```python
from build123d import *

# Parameters (mm, degrees)
SKETCH1_R               = 94.996
SKETCH1_R_2             = 53.975
TOP_OF_HATCH_DEPTH      = 3.302
SKETCH2_R               = 94.996
SKETCH2_R_2             = 89.789
HATCH_BODY_DEPTH        = 259.08
SKETCH3_R               = 13.335
CHARGE_TUBE_HOLES_DEPTH = 263.382
SKETCH4_R               = 3.81
BOLT_HOLES_DEPTH        = 263.382
SKETCH_5_R              = 5.08
ANTENNA_HOLES_DEPTH     = 263.382
SKETCH5_R               = 3.81
SKETCH5_R_2             = 3.175
INNER_SCREW_HOLES_DEPTH = 263.382
SKETCH8_R               = 1.397
CUT_EXTRUDE1_DEPTH      = 190.992
CUT_EXTRUDE4_DEPTH      = 263.3820001


with BuildPart() as part:
    # Sketch1 → Top of Hatch (new body)
    with BuildSketch(Plane(origin=(0, 0, 0), x_dir=(1, 0, 0), z_dir=(0, 1, 0))):
        Circle(SKETCH1_R)
        Circle(SKETCH1_R_2, mode=Mode.SUBTRACT)
    extrude(amount=TOP_OF_HATCH_DEPTH)

    # Sketch2 → Hatch Body (add)
    with BuildSketch(Plane(origin=(0, 3.302, 0), x_dir=(1, 0, 0), z_dir=(0, 1, 0))):
        Circle(SKETCH2_R)
        Circle(SKETCH2_R_2, mode=Mode.SUBTRACT)
    extrude(amount=HATCH_BODY_DEPTH)

    # Sketch3 → Charge Tube Holes (cut, through all)
    with BuildSketch(Plane.XZ):
        with Locations((-76.454, 0)):
            Circle(SKETCH3_R)
        with Locations((76.454, 0)):
            Circle(SKETCH3_R)
    extrude(amount=-CHARGE_TUBE_HOLES_DEPTH, mode=Mode.SUBTRACT)

    # Sketch4 → Bolt Holes (cut, through all)
    with BuildSketch(Plane.XZ):
        with Locations((-38.1, -65.991135768)):
            Circle(SKETCH4_R)
        with Locations((-38.1, 65.991135768)):
            Circle(SKETCH4_R)
        with Locations((38.1, 65.991135768)):
            Circle(SKETCH4_R)
        with Locations((38.1, -65.991135768)):
            Circle(SKETCH4_R)
    extrude(amount=-BOLT_HOLES_DEPTH, mode=Mode.SUBTRACT)

    # Sketch 5 → Antenna Holes (cut, through all)
    with BuildSketch(Plane.XZ):
        with Locations((-26.112352144, 57.324838678)):
            Circle(SKETCH_5_R)
        with Locations((9.193647856, 61.033450854)):
            Circle(SKETCH_5_R)
    extrude(amount=-ANTENNA_HOLES_DEPTH, mode=Mode.SUBTRACT)

    # Sketch5 → Inner Screw Holes (cut, through all)
    with BuildSketch(Plane.XZ):
        with Locations((58.42, 0)):
            Circle(SKETCH5_R)
        with Locations((-58.42, 0)):
            Circle(SKETCH5_R)
        with Locations((39.878, 41.91)):
            Circle(SKETCH5_R_2)
        with Locations((-39.878, 41.91)):
            Circle(SKETCH5_R_2)
        with Locations((39.878, -41.91)):
            Circle(SKETCH5_R_2)
        with Locations((-39.878, -41.91)):
            Circle(SKETCH5_R_2)
    extrude(amount=-INNER_SCREW_HOLES_DEPTH, mode=Mode.SUBTRACT)

    # Sketch8 → Cut-Extrude1 (cut, through all)
    with BuildSketch(Plane(origin=(94.996, 0, 0), x_dir=(0, 0, -1), z_dir=(1, 0, 0))):
        with Locations((14.351, 198.882)):
            Circle(SKETCH8_R)
        with Locations((-14.351, 198.882)):
            Circle(SKETCH8_R)
    extrude(amount=-CUT_EXTRUDE1_DEPTH, mode=Mode.SUBTRACT)

    # Sketch12 → Cut-Extrude4 (cut, through all)
    with BuildSketch(Plane.XZ):
        with BuildLine():
            Line((-94.996, 0), (94.996, 0))
            ThreePointArc((94.996, 0), (0, -94.996), (-94.996, 0))
        make_face()
    extrude(amount=-CUT_EXTRUDE4_DEPTH, mode=Mode.SUBTRACT)


solid = part.part
```
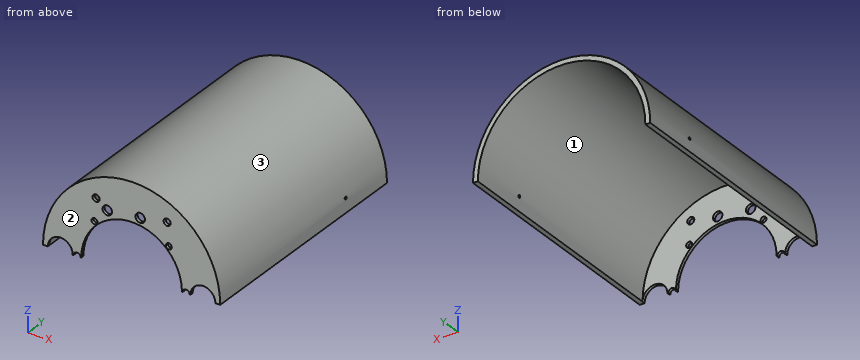
Read the model definition and answer for the solid it produces. Units are mm, in the model's axes. Face numbers are marked on the shaded views. Coordinates: 2 decimals unless noted, no trailing zeros. Order: outer loops, then holes, each group sorted by start corner. A loop starts at its lowest first (then second) coordinate and runs counter-clockwise, first axis right, second up. Notation, with made-up numbers: (20, 63.25) - (45, 63.25) arc R22 ccw to (45, 91.25) - close; hole circle Ø7 at (72.25, 50). An arc over 180 degrees is marked (long way). Answer as a JSON object with one key per item and string values. Group by question number.
Item 1: The mould has two halves that part along X. Classify the marked faces 1, 2 and 3: +X half, -X half, draft (parallel to the pull), parting line (faces both ways), or undercut.
Item 2: Section D-D (y = 117) is taken. Give the vertices of the cut face in (x, z).
Item 3: Section B-B (x = 0) is taken. Give the vertices of the cut face in (y, z) (3 decimals), plus the area to 3 significant figures.
Item 4: Section C-C (z = 75.5) is taken. Give the vertices of the cut face in (x, y).
Item 5: Flat-ended cylindrical pins translate along their axes: P1, Ø5, axis at y = 139.5, z = 50, coming from the -X side; P2, Ø10, axis at y = 163.5, z = 44, coming from the +X side; P3, Ø6, axis at x = -31.5, z = 80, coming from the -Y side; P4, Ø10, axis at x = 21.5, y = 187.5, coming from the +Z side. Find the tip coordinate at first contact, or state that the pin passes through.
Item 6: Consider probe 1 along X at (y, z) = (2, 41); probe 2 along X at (y, z) = (162.5, 46.5); probe 3 along X at (y, z) = (120.5, 7). Determine where each line is inside the solid, lowest interval first. Write a range as from..to.
Item 7: Section A-A (z = 35) is taken. Give the vertices of the cut face in (x, y), plus the area to 3 significant figures.
Results are:
{
 "1": {"face 1": "undercut", "face 2": "draft", "face 3": "parting line"},
 "2": {"outline": "(-95, 0) - (-89.79, 0) arc R89.79 cw to (89.79, 0) - (95, 0) arc R95 ccw to start"},
 "3": {"outline": "(0, 53.975) - (3.302, 53.975) - (3.302, 89.789) - (262.382, 89.789) - (262.382, 94.996) - (0, 94.996) - close", "area": "1,480 mm^2"},
 "4": {"outline": "(-57.65, 0) - (57.65, 0) - (57.65, 262.38) - (48.6, 262.38) - (48.6, 3.3) - (-48.6, 3.3) - (-48.6, 262.38) - (-57.65, 262.38) - close"},
 "5": {"P1": "stops at x = -82.27", "P2": "stops at x = 86.62", "P3": "stops at y = 0", "P4": "stops at z = 93.55"},
 "6": {"probe 1": "x = -85.69..-42.92, -36.84..-35.1, 35.1..36.84, 42.92..85.69", "probe 2": "x = -82.84..-76.81, 76.81..82.84", "probe 3": "x = -94.74..-89.52, 89.52..94.74"},
 "7": {"outline": "(-88.31, 0) - (-41.09, 0) - (-41.09, 3.3) - (-82.69, 3.3) - (-82.69, 262.38) - (-88.31, 262.38) - close; (41.09, 0) - (88.31, 0) - (88.31, 262.38) - (82.69, 262.38) - (82.69, 3.3) - (41.09, 3.3) - close", "area": "3,230 mm^2"}
}
